```python
from build123d import *

# Parameters (mm, degrees)
SKETCH1_R           = 35
SKETCH1_R_2         = 25
BOSS_EXTRUDE1_DEPTH = 50
SKETCH2_R           = 35
BOSS_EXTRUDE2_DEPTH = 12
SKETCH3_R           = 7
CUT_EXTRUDE1_DEPTH  = 12
CHAMFER1_SIZE       = 5


with BuildPart() as part:
    # Sketch1 → Boss-Extrude1 (new body)
    with BuildSketch(Plane.XY):
        Circle(SKETCH1_R)
        Circle(SKETCH1_R_2, mode=Mode.SUBTRACT)
    extrude(amount=BOSS_EXTRUDE1_DEPTH)

    # Sketch2 → Boss-Extrude2 (add)
    with BuildSketch(Plane.XY):
        with BuildLine():
            Line((-29.647715243, -46.325079394), (-88.936024476, -10.715763573))
            ThreePointArc((-88.936024476, -10.715763573), (-95, 0), (-88.936024476, 10.715763573))
            Line((-88.936024476, 10.715763573), (-29.647715243, 46.325079394))
            ThreePointArc((-29.647715243, 46.325079394), (0, 55), (29.647715243, 46.325079394))
            Line((29.647715243, 46.325079394), (88.936024476, 10.715763573))
            ThreePointArc((88.936024476, 10.715763573), (95, 0), (88.936024476, -10.715763573))
            Line((88.936024476, -10.715763573), (29.647715243, -46.325079394))
            ThreePointArc((29.647715243, -46.325079394), (0, -55), (-29.647715243, -46.325079394))
        make_face()
        Circle(SKETCH2_R, mode=Mode.SUBTRACT)
    extrude(amount=BOSS_EXTRUDE2_DEPTH)

    # Sketch3 → Cut-Extrude1 (cut)
    with BuildSketch(Plane(origin=(0, 0, 0), x_dir=(-1, 0, 0), z_dir=(0, 0, -1))):
        with Locations((-82.5, 0)):
            Circle(SKETCH3_R)
        with Locations((82.5, 0)):
            Circle(SKETCH3_R)
    extrude(amount=-CUT_EXTRUDE1_DEPTH, mode=Mode.SUBTRACT)

    # Chamfer1
    chamfer1_edges = [part.edges().sort_by_distance(p)[0] for p in [
        (-35, 0, 12),
    ]]
    chamfer(chamfer1_edges, length=CHAMFER1_SIZE)


solid = part.part
```
Geometry check sheet. Reference: the model listing, model coordinates, mm. A direction names the side the tool comes from. Give positions to 0.01 mm unless a question says otherwise; leave off trailing zeros. Write each loop counter-clockwise with the first axis right and the second up, starting at its lowest first coordinate (ties: lowest second). Pieces come first, ordered by that corner, then holes.
1) Material ranges on L1, parallel to X at y = 10.5, z = 16; L2, parallel to X at y = -16, z = 43.5; L3, parallel to Z at x = -3.5, y = 45.5, recorded low to high.
2) Gauge pin test, flat ends, axial feed: pin 1 (5 mm diameter, centred on y = 12, z = 29.5, fed in from +X); pin 2 (8 mm diameter, centred on x = 14.5, z = 18, fed in from -Y); pin 3 (6 mm diameter, centred on x = -14, y = -42.5, fed in from +Z). Record the tip position at first contact, or that the pin passes through.
3) Release check for a two-part mould opening along Y. For faces 3 (the cylindrical face through (-95, 0, 6)), 4 (the flat face through (-58.88, -28.77, 5.92)), 5 (the cylindrical face through (-75.507, 0.308, 5.916)) record: pulls with the +Y half, pulls with the -Y half, needs draft (parallel to the pull), parting line crosses it, or undercut.
4) Section check A-A, the plane x = 0. Record the boundary of the cut face in (y, z), and give its area (4 significant figures).
5) Section check D-D, the plane y = 44. Record the boundary of the cut face in (x, z).
6) Section check B-B, the plane z = 39.5. Record the boundary of the cut face in (x, y).
7) Section check C-C, the plane x = 82.5. Record the boundary of the cut face in (y, z).
8) Access from +Z, -Z, +X, -X, +Y, -Y to the whole of each face (thin tool, end or side, straight path). Record for faces 1 (the flat face through (-24, 8, 50)), 2 (the flat face through (-41, 1, 12)).
Computed:
1. L1: x = -34.43 to -22.69, 22.69 to 34.43
1. L2: x = -31.13 to -19.21, 19.21 to 31.13
1. L3: z = 0 to 12
2. pin 1: stops at x = 33.69
2. pin 2: stops at y = -35.4
2. pin 3: stops at z = 12
3. face 3: parting line crosses it
3. face 4: pulls with the -Y half
3. face 5: undercut
4. outline: (-55, 0) - (-25, 0) - (-25, 50) - (-35, 50) - (-35, 17) - (-40, 12) - (-55, 12) - close; (25, 0) - (55, 0) - (55, 12) - (40, 12) - (35, 17) - (35, 50) - (25, 50) - close
4. area: 1,505 mm2
5. outline: (-33.52, 0) - (33.52, 0) - (33.52, 12) - (-33.52, 12) - close
6. outline: circle Ø70 at (0, 0); hole circle Ø50 at (0, 0)
7. outline: (-14.58, 0) - (-7, 0) - (-7, 12) - (-14.58, 12) - close; (7, 0) - (14.58, 0) - (14.58, 12) - (7, 12) - close
8. face 1: +Z, +X, -X, +Y, -Y
8. face 2: +Z
